```python
from build123d import *

# Parameters (mm, degrees)
BOSS_EXTRUDE1_DEPTH = 25
SKETCH2_R           = 13.5
CUT_EXTRUDE1_DEPTH  = 25
SKETCH3_R           = 13.5
CUT_EXTRUDE2_DEPTH  = 25
SKETCH4_R           = 13.5
SKETCH4_R_2         = 10
BOSS_EXTRUDE2_DEPTH = 5
BOSS_EXTRUDE3_START = -15
SKETCH5_R           = 13.5
SKETCH5_R_2         = 10
BOSS_EXTRUDE3_DEPTH = 15
CUT_EXTRUDE3_DEPTH  = 10
SKETCH7_R           = 13.468633883
BOSS_EXTRUDE4_DEPTH = 3
CUT_EXTRUDE4_START  = -16.6
CUT_EXTRUDE4_DEPTH  = 16.6
FILLET1_R           = 10
FILLET2_R           = 10
FILLET4_R           = 8


# Some blends are built 0.0001 mm under size
with BuildPart() as part:
    # Sketch1 → Boss-Extrude1 (new body)
    with BuildSketch(Plane.XY):
        with BuildLine():
            Line((-154.944852941, 25), (-4.944852941, 25))
            ThreePointArc((-4.944852941, 25), (20.055147059, 0), (-4.944852941, -25))
            Line((-4.944852941, -25), (-154.944852941, -25))
            ThreePointArc((-154.944852941, -25), (-179.944852941, 0), (-154.944852941, 25))
        make_face()
    extrude(amount=BOSS_EXTRUDE1_DEPTH)

    # Sketch2 → Cut-Extrude1 (cut)
    with BuildSketch(Plane.XY.offset(25)):
        with Locations((-4.944852941, 0)):
            Circle(SKETCH2_R)
    extrude(amount=-CUT_EXTRUDE1_DEPTH, mode=Mode.SUBTRACT)

    # Sketch3 → Cut-Extrude2 (cut)
    with BuildSketch(Plane.XY.offset(25)):
        with Locations((-154.944852941, 0)):
            Circle(SKETCH3_R)
    extrude(amount=-CUT_EXTRUDE2_DEPTH, mode=Mode.SUBTRACT)

    # Sketch4 → Boss-Extrude2 (add)
    with BuildSketch(Plane.XY.offset(25)):
        with Locations((-4.944852941, 0)):
            Circle(SKETCH4_R)
        with Locations((-4.944852941, 0)):
            Circle(SKETCH4_R_2, mode=Mode.SUBTRACT)
    extrude(amount=-BOSS_EXTRUDE2_DEPTH)

    # Sketch5 → Boss-Extrude3 (add)
    with BuildSketch(Plane(origin=(0, 0, 0), x_dir=(-1, 0, 0), z_dir=(0, 0, -1)).offset(BOSS_EXTRUDE3_START)):
        with Locations(Location((4.944852941, 0, 0), (0, 0, 180))):
            Circle(SKETCH5_R)
        with Locations(Location((4.944852941, 0, 0), (0, 0, 180))):
            Circle(SKETCH5_R_2, mode=Mode.SUBTRACT)
    extrude(amount=BOSS_EXTRUDE3_DEPTH)

    # Sketch6 → Cut-Extrude3 (cut)
    with BuildSketch(Plane(origin=(0, 0, 0), x_dir=(-1, 0, 0), z_dir=(0, 0, -1))):
        with BuildLine():
            Line((4.944852941, 25), (34.850592548, 25))
            Line((34.850592548, 25), (34.850592548, -25))
            Line((34.850592548, -25), (4.944852941, -25))
            ThreePointArc((4.944852941, -25), (-20.055147059, 0), (4.944852941, 25))
        make_face()
    extrude(amount=-CUT_EXTRUDE3_DEPTH, mode=Mode.SUBTRACT)


with BuildPart() as body_2:
    # Sketch7 → Boss-Extrude4 (new body)
    with BuildSketch(Plane.XY.offset(25)):
        with Locations((-154.944852941, 0)):
            Circle(SKETCH7_R)
    extrude(amount=-BOSS_EXTRUDE4_DEPTH)


with BuildPart() as cut_extrude4_tool:
    # Sketch9 → Cut-Extrude4 (new body)
    with BuildSketch(Plane.XY.offset(25).offset(CUT_EXTRUDE4_START)):
        with BuildLine():
            Line((-96.084788757, 25), (-96.084788757, -25))
            Line((-96.084788757, -25), (-154.944852941, -25))
            ThreePointArc((-154.944852941, -25), (-179.944852941, 0), (-154.944852941, 25))
            Line((-154.944852941, 25), (-96.084788757, 25))
        make_face()
    extrude(amount=CUT_EXTRUDE4_DEPTH)


with BuildPart() as part_1:
    add(part.part)

    # Cut-Extrude4: cut by cut_extrude4_tool
    add(cut_extrude4_tool.part, mode=Mode.SUBTRACT)

    # Fillet1
    fillet1_edges = [part_1.edges().sort_by_distance(p)[0] for p in [
        (-96.084788757, 0, 25),
    ]]
    fillet(fillet1_edges, radius=FILLET1_R)

    # Fillet2
    fillet2_edges = [part_1.edges().sort_by_distance(p)[0] for p in [
        (-34.850592548, 0, 0),
    ]]
    fillet(fillet2_edges, radius=FILLET2_R - 0.0001)  # a hair under: the kernel refuses the full size

    # Fillet4
    # the kernel refuses this fillet: 8 mm, written as the material it takes off along each edge
    with BuildSketch(Plane(origin=(-4.944852941, 0, 25), x_dir=(0, 1, 0), z_dir=(-1, 0, 0))) as fillet4_piece_1:
        with BuildLine():
            CenterArc((25 - FILLET4_R, FILLET4_R), FILLET4_R, 270, 90)
            Line((25 - FILLET4_R, 0), (25, 0))
            Line((25, 0), (25, FILLET4_R))
        make_face()
    revolve(axis=Axis((-4.944852941, 0, 25), (0, 0, -1)), revolution_arc=180, mode=Mode.SUBTRACT)
    with BuildSketch(Plane(origin=(-86.084788757, 25, 25), x_dir=(0, -1, 0), z_dir=(1, 0, 0))) as fillet4_piece_2:
        with BuildLine():
            CenterArc((FILLET4_R, FILLET4_R), FILLET4_R, 180, 90)
            Line((0, FILLET4_R), (0, 0))
            Line((0, 0), (FILLET4_R, 0))
        make_face()
    extrude(amount=81.139935816, mode=Mode.SUBTRACT)
    with BuildSketch(Plane(origin=(-154.944852941, 0, 0), x_dir=(1, 0, 0), z_dir=(0, -1, 0))) as fillet4_piece_3:
        with BuildLine():
            CenterArc((13.5 + FILLET4_R, FILLET4_R), FILLET4_R, 180, 90)
            Line((13.5, FILLET4_R), (13.5, 0))
            Line((13.5, 0), (13.5 + FILLET4_R, 0))
        make_face()
    revolve(axis=Axis((-154.944852941, 0, 0), (0, 0, 1)), mode=Mode.SUBTRACT)
    with BuildSketch(Plane(origin=(-4.944852941, 0, 25), x_dir=(1, 0, 0), z_dir=(0, -1, 0))) as fillet4_piece_4:
        with BuildLine():
            CenterArc((17.416198487, -8), FILLET4_R, 90, 67.975687163)
            Line((10, -5), (10, 0))
            Line((10, 0), (17.416198487, 0))
        make_face()
    revolve(axis=Axis((-4.944852941, 0, 25), (0, 0, 1)), mode=Mode.SUBTRACT)
    with BuildSketch(Plane(origin=(-44.850492548, -25, 0), x_dir=(0, 0, 1), z_dir=(-1, 0, 0))) as fillet4_piece_5:
        with BuildLine():
            CenterArc((FILLET4_R, FILLET4_R), FILLET4_R, 180, 90)
            Line((0, FILLET4_R), (0, 0))
            Line((0, 0), (FILLET4_R, 0))
        make_face()
    extrude(amount=110.094360393, mode=Mode.SUBTRACT)
    with BuildSketch(Plane(origin=(-154.944852941, 0, 0), x_dir=(0, -1, 0), z_dir=(1, 0, 0))) as fillet4_piece_6:
        with BuildLine():
            CenterArc((25 - FILLET4_R, -FILLET4_R), FILLET4_R, 0, 90)
            Line((25, -FILLET4_R), (25, 0))
            Line((25, 0), (25 - FILLET4_R, 0))
        make_face()
    revolve(axis=Axis((-154.944852941, 0, 0), (0, 0, -1)), revolution_arc=180, mode=Mode.SUBTRACT)
    with BuildSketch(Plane(origin=(-96.084788757, 25, 8.4), x_dir=(0, -1, 0), z_dir=(0, 0, 1)), Plane(origin=(-96.084788757, -25, 8.4), x_dir=(1, 0, 0), z_dir=(0, 0, 1))) as fillet4_piece_7:
        with BuildLine():
            CenterArc((FILLET4_R, FILLET4_R), FILLET4_R, 180, 90)
            Line((0, FILLET4_R), (0, 0))
            Line((0, 0), (FILLET4_R, 0))
        make_face()
    extrude(amount=6.6, mode=Mode.SUBTRACT)
    with BuildSketch(Plane(origin=(-86.084788757, 25, 15), x_dir=(-1, 0, 0), z_dir=(0, 0, -1))) as fillet4_piece_8:
        with BuildLine():
            CenterArc((10 - FILLET4_R, -FILLET4_R), FILLET4_R, 0, 90)
            Line((10 - FILLET4_R, 0), (10, 0))
            Line((10, 0), (10, -FILLET4_R))
        make_face()
    revolve(axis=Axis((-86.084788757, 25, 15), (0, 1, 0)), revolution_arc=90, mode=Mode.SUBTRACT)
    with BuildSketch(Plane(origin=(-4.944852941, -25, 25), x_dir=(0, 0, -1), z_dir=(-1, 0, 0))) as fillet4_piece_9:
        with BuildLine():
            CenterArc((FILLET4_R, -FILLET4_R), FILLET4_R, 90, 90)
            Line((0, -FILLET4_R), (0, 0))
            Line((0, 0), (FILLET4_R, 0))
        make_face()
    extrude(amount=81.139935816, mode=Mode.SUBTRACT)
    with BuildSketch(Plane(origin=(-86.084788757, -25, 15), x_dir=(-1, 0, 0), z_dir=(0, 0, -1))) as fillet4_piece_10:
        with BuildLine():
            CenterArc((10 - FILLET4_R, FILLET4_R), FILLET4_R, 270, 90)
            Line((10, FILLET4_R), (10, 0))
            Line((10, 0), (10 - FILLET4_R, 0))
        make_face()
    revolve(axis=Axis((-86.084788757, -25, 15), (0, 1, 0)), revolution_arc=90, mode=Mode.SUBTRACT)
    with BuildSketch(Plane(origin=(-154.944852941, 25, 0), x_dir=(0, -1, 0), z_dir=(1, 0, 0))) as fillet4_piece_11:
        with BuildLine():
            CenterArc((FILLET4_R, -FILLET4_R), FILLET4_R, 90, 90)
            Line((0, -FILLET4_R), (0, 0))
            Line((0, 0), (FILLET4_R, 0))
        make_face()
    extrude(amount=110.094360393, mode=Mode.SUBTRACT)
    with BuildSketch(Plane(origin=(-44.850492548, 25, 9.9999), x_dir=(0, 0, -1), z_dir=(-1, 0, 0))) as fillet4_piece_12:
        with BuildLine():
            CenterArc((9.9999 - FILLET4_R, FILLET4_R), FILLET4_R, 270, 90)
            Line((9.9999 - FILLET4_R, 0), (9.9999, 0))
            Line((9.9999, 0), (9.9999, FILLET4_R))
        make_face()
    revolve(axis=Axis((-44.850492548, 25, 9.9999), (0, -1, 0)), revolution_arc=90, mode=Mode.SUBTRACT)
    with BuildSketch(Plane(origin=(-44.850492548, -25, 9.9999), x_dir=(0, 0, -1), z_dir=(-1, 0, 0))) as fillet4_piece_13:
        with BuildLine():
            CenterArc((9.9999 - FILLET4_R, -FILLET4_R), FILLET4_R, 0, 90)
            Line((9.9999, -FILLET4_R), (9.9999, 0))
            Line((9.9999, 0), (9.9999 - FILLET4_R, 0))
        make_face()
    revolve(axis=Axis((-44.850492548, -25, 9.9999), (0, -1, 0)), revolution_arc=90, mode=Mode.SUBTRACT)
    with BuildSketch(Plane(origin=(-34.850592548, -25, 9.9999), x_dir=(-1, 0, 0), z_dir=(0, 0, 1)), Plane(origin=(-34.850592548, 25, 9.9999), x_dir=(0, -1, 0), z_dir=(0, 0, 1))) as fillet4_piece_14:
        with BuildLine():
            CenterArc((FILLET4_R, -FILLET4_R), FILLET4_R, 90, 90)
            Line((0, -FILLET4_R), (0, 0))
            Line((0, 0), (FILLET4_R, 0))
        make_face()
    extrude(amount=0.0001, mode=Mode.SUBTRACT)


with BuildPart() as body_2_1:
    add(body_2.part)

    # Cut-Extrude4: cut by cut_extrude4_tool
    add(cut_extrude4_tool.part, mode=Mode.SUBTRACT)


solid = part_1.part
```
The listing builds one solid part. Answer for the finished solid, in the listing's coordinates (mm). A direction names the side the tool comes from. Coordinates: 2 decimals unless noted, no trailing zeros. Write each loop counter-clockwise with the first axis right and the second up, starting at its lowest first coordinate (ties: lowest second). Pieces come first, ordered by that corner, then holes. Notation, with made-up numbers: (89, 56) -> (122, 56) arc R21 ccw to (122, 90) -> close; hole circle Ø9 at (16.5, 7.5). An arc over 180 degrees is marked (long way). Write each question's results on one line, items separated by ' | '. Start each with the question number.
1) A cutting plane is placed at B-B (x = -72). Determine the outline of the cut face in (y, z).
2) A cutting plane is placed at A-A (y = 0). Count the separate pieces of the cut face and the enclosed holes in it, then the cut area to 3 significant figures.
3) A cutting plane is placed at C-C (x = -100). Determine the outline of the cut face in (y, z), then the cut area to 3 significant figures.
4) A tool of negligible diameter and unlimited length cuts with its end or side. For faces 1 (the cylindrical face through (-93.8, -22.6, 11.7)), 2 (the flat face through (-96.085, 0, 12)), 3 (the cylindrical face through (-93.7, 22.7, 11.7)), from which of +Z, -Z, +X, -X, +Y, -Y can it reach the whole face along a straight path? Write none if from no direction.
5) Straight lines are drawn through the part: probe 1 along X at (y, z) = (-7, 7); probe 2 along Y at (x, z) = (3, 23.5); probe 3 along Z at (x, y) = (-13, 7.5). For each, find the intervals that lie inside material, in ascending order.
6) Flat-ended cylindrical pins translate along their axes: pin 1 Ø6 at (y, z) = (-10.5, 5.5) entering from -X; pin 2 Ø8 at (y, z) = (8, 8.5) entering from +X; pin 3 Ø23 at (x, y) = (-4.94, 0) entering from -Z; pin 4 Ø6 at (x, y) = (-64.5, -11) entering from -Z. Find the tip coordinate at first contact, or state that the pin passes through.
Values follow:
1) outline: (-25, 8) arc R8 ccw to (-17, 0) -> (17, 0) arc R8 ccw to (25, 8) -> (25, 17) arc R8 ccw to (17, 25) -> (-17, 25) arc R8 ccw to (-25, 17) -> close
2) separate pieces: 3 | enclosed holes: 0 | area: 2,380 mm²
3) outline: (-25, 8) arc R8 ccw to (-17, 0) -> (17, 0) arc R8 ccw to (25, 8) -> (25, 8.4) -> (-25, 8.4) -> close | area: 393 mm²
4) face 1: +Z, -X, -Y | face 2: +Z, -X, +Y, -Y | face 3: +Z, -X, +Y
5) probe 1: -178.88 to -166.56, -143.33 to -35.31 | probe 2: -20.15 to -9.98, 9.98 to 20.15 | probe 3: 10 to 15, 20 to 21.79
6) pin 1: x = -178.6 | pin 2: x = 19.68 | pin 3: z = 10 | pin 4: z = 0
